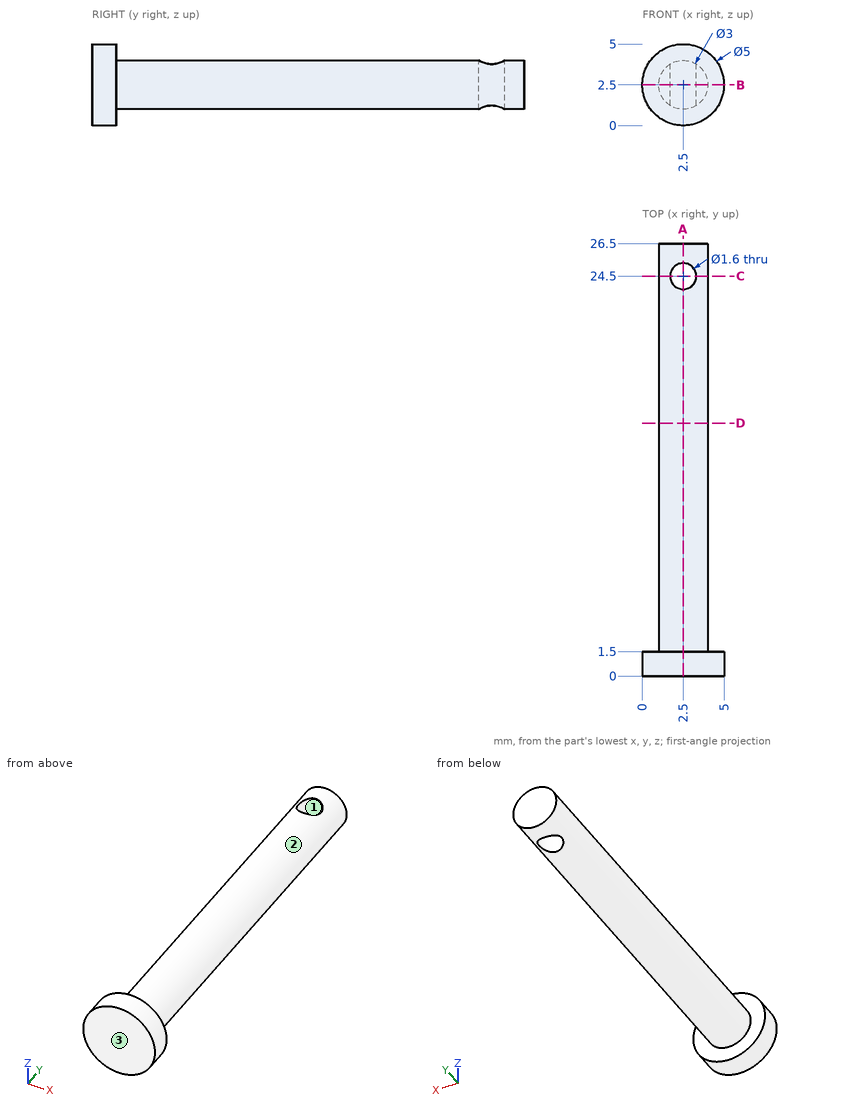
The figure shows three views and two pictorial views of one solid part (mm, origin at its lowest corner). Answer the questions. Round coordinates to 2 decimals unless told otherwise and drop trailing zeros. Loops run counter-clockwise (first coordinate to the right, second up) from the corner with the lowest first, then second, coordinate; pieces in that order, holes last. Notation, with made-up numbers: M 24,22 L 71,22 A32 cw 71,58 Z; hole C 66.25,-17 d6. An arc over 180 degrees is marked long. Use CSV: the item, a comma, the result in double quotes.
Q1. Section D-D, the plane y = 15.5 is taken. Determine the outline of the cut face in (x, z), then the cut area to 3 significant figures.
Determined:
outline,"C 2.5,2.5 d3"
area,"7.07 mm2"
Q2. Each of these flat-tipped pins is pushed along its axis until it touches: pin 1 (1 mm diameter, centred on x = 4.5, z = 2, fed in from +Y); pin 2 (1.3 mm diameter, centred on x = 2.5, y = 24.5, fed in from +Z); pin 3 (1.5 mm diameter, centred on y = 22, z = 1, fed in from -X); pin 4 (3 mm diameter, centred on y = 19.5, z = 2, fed in from -X). Where does it stop, or does it pass through?
Determined:
pin 1,"y = 1.5"
pin 2,"through"
pin 3,"x = 1.2"
pin 4,"x = 1"
Q3. The mould has two halves that part along X. Classify the marked faces 1, 2 and 3: pulls with the +X half, pulls with the -X half, needs draft (parallel to the pull), parting line crosses it, or undercut.
Determined:
face 1,"undercut"
face 2,"parting line crosses it"
face 3,"needs draft"
Q4. Section A-A, the plane x = 2.5 is taken. Determine the outline of the cut face in (y, z).
Determined:
outline,"M 0,0 L 1.5,0 L 1.5,1 L 23.7,1 L 23.7,4 L 1.5,4 L 1.5,5 L 0,5 Z; M 25.3,1 L 26.5,1 L 26.5,4 L 25.3,4 Z"
Q5. Consider L1, parallel to X at y = 25, z = 3.5; L2, parallel to X at y = 24.5, z = 1.9; L3, parallel to X at y = 5, z = 2.6. Determine where each line is inside the solid, lowest interval first.
Determined:
L1,"1.38 to 1.88, 3.12 to 3.62"
L2,"1.13 to 1.7, 3.3 to 3.87"
L3,"1 to 4"
Q6. Section B-B, the plane z = 2.5 is taken. Determine the outline of the cut face in (x, y).
Determined:
outline,"M 0,0 L 5,0 L 5,1.5 L 4,1.5 L 4,26.5 L 1,26.5 L 1,1.5 L 0,1.5 Z; hole C 2.5,24.5 d1.6"
Q7. Section C-C, the plane y = 24.5 is taken. Determine the outline of the cut face in (x, z), then the cut area to 3 significant figures.
Determined:
outline,"M 1.7,1.23 L 1.7,3.77 A1.5 ccw Z; M 3.3,1.23 A1.5 ccw 3.3,3.77 Z"
area,"2.51 mm2"
